CAD build for the part. Positions are in the model's coordinates, mm. Face numbers are marked on the shaded views. A direction names the side the tool comes from. Coordinates: 2 decimals unless noted, no trailing zeros. Loops run counter-clockwise (first coordinate to the right, second up) from the corner with the lowest first, then second, coordinate; pieces in that order, holes last. Notation, with made-up numbers: (-15.5, -22) -> (39.5, -22) arc R25 cw to (39.5, 15) -> close; hole circle Ø7 at (-36, -29). An arc over 180 degrees is marked (long way). Answer as CSV lines item,"result". Start each with the question number.
```python
from build123d import *

# Parameters (mm, degrees)
CHAMFER_1_SIZE = 1
SKETCH_2_W     = 3
SKETCH_2_H     = 41.75


with BuildPart() as part:
    # Эскиз1 → Повернуть1 (revolve)
    with BuildSketch(Plane.XY, mode=Mode.PRIVATE) as revolve_1_sk:
        Polygon((31, 35), (31, 45), (19, 45), (19, 50), (0, 50), (0, 40), (24, 40), (24, 35), align=None)
    revolve(revolve_1_sk.sketch.rotate(Axis((0, 0, 0), (1, 0, 0)), 90), axis=Axis((0, 0, 0), (1, 0, 0)))

    # Фаска1
    chamfer_1_edges = [part.edges().sort_by_distance(p)[0] for p in [
        (31, 0, -45),
        (0, 0, -40),
        (0, 0, -50),
        (19, 0, -50),
    ]]
    chamfer(chamfer_1_edges, length=CHAMFER_1_SIZE)

    # Эскиз2 → Вырез-Повернуть1 (revolve, cut)
    with BuildSketch(Plane.XY, mode=Mode.PRIVATE) as cut_revolve_1_sk:
        with Locations((4.5, 20.875)):
            Rectangle(SKETCH_2_W, SKETCH_2_H)
    revolve(cut_revolve_1_sk.sketch.rotate(Axis((0, 0, 0), (1, 0, 0)), 270), axis=Axis((0, 0, 0), (1, 0, 0)), mode=Mode.SUBTRACT)


solid = part.part
```
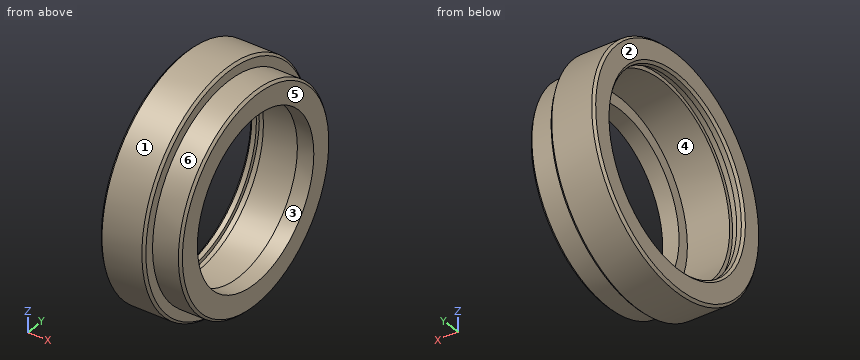
Q1. Probe probe 1 along Y at (x, z) = (2, 0); probe 2 along Y at (x, z) = (29.25, 0); probe 3 along Z at (x, y) = (2, 4). List the from-to ranges inside material, lowest first. Write a range as from..to.
Q2. Saw through at D-D (x = 8.5). List the corners of the cut face in (y, z).
Q3. Pin check, flat tips, straight feed: pin 1 Ø1 at (y, z) = (-36, 10.5) entering from -X; pin 2 Ø10 at (x, z) = (20, 35.5) entering from +Y; pin 3 Ø12 at (x, y) = (6, 36.5) entering from -Z. Stop position of each tip, or through.
Q4. Which spindle directions (+Z, -Z, +X, -X, +Y, -Y) get a long thin tool onto all of the face, cutting with end or side? Do the marked faces 4, 5 and 6. Say none if no direction does.
Q5. Saw through at C-C (x = 25.5). List the corners of the cut face in (y, z).
Q6. Two-plate mould, pull along Z, no slides. Class the marked faces 1, 2 and 3: pulls with the +Z half, pulls with the -Z half, needs draft (parallel to the pull), parting line crosses it, or undercut.
Ans:
1,probe 1,"y = -50..-40, 40..50"
1,probe 2,"y = -45..-35, 35..45"
1,probe 3,"z = -49.84..-39.8, 39.8..49.84"
2,outline,"circle Ø100 at (0, 0); hole circle Ø80 at (0, 0)"
3,pin 1,"stops at x = 24"
3,pin 2,"stops at y = 39.3"
3,pin 3,"stops at z = -39.62"
4,face 4,"-X"
4,face 5,"+Z, -Z, +X, +Y, -Y"
4,face 6,"+X"
5,outline,"circle Ø90 at (0, 0); hole circle Ø70 at (0, 0)"
6,face 1,"parting line crosses it"
6,face 2,"needs draft"
6,face 3,"undercut"
